Autodesk Inventor part; units mm, degrees
ref_plane "YZ Plane" through (0, 0, 0) normal (1, 0, 0) x (0, 1, 0)
ref_plane "XZ Plane" through (0, 0, 0) normal (0, 1, 0) x (-1, 0, 0)
ref_plane "XY Plane" through (0, 0, 0) normal (0, 0, 1) x (1, 0, 0)
sketch "スケッチ2" plane through (0, 0, 0) normal (0, 1, 0) x (-1, 0, 0)
  line L0 (-30, 15) -> (30, 15)
  line L1 (30, 15) -> (30, -15)
  line L2 (30, -15) -> (-30, -15)
  line L3 (-30, -15) -> (-30, 15)
  line L4 (-30, 15) -> (30, -15) construction
  line L5 (30, 15) -> (-30, -15) construction
  line L6 (27.7, -12.7) -> (27.7, 12.7)
  line L7 (27.7, 12.7) -> (-27.7, 12.7)
  line L8 (-27.7, 12.7) -> (-27.7, -12.7)
  line L9 (-27.7, -12.7) -> (27.7, -12.7)
  point P0 (0, 0)
  dimension "d0" = 60
  dimension "d1" = 30
  dimension "d2" = 2.3
extrude "押し出し1" add sketch "スケッチ2" along normal mid plane 100
sketch "スケッチ3" plane through (30, -50, -15) normal (1, 0, 0) x (0, 0, -1)
  circle A0 centre (-15, 30) radius 6
  point P0 (-15, 50)
  dimension "d5" = 12
  dimension "d6" = 20
extrude "押し出し2" cut sketch "スケッチ3" against normal blind 60
properties part number "車軸受け1"
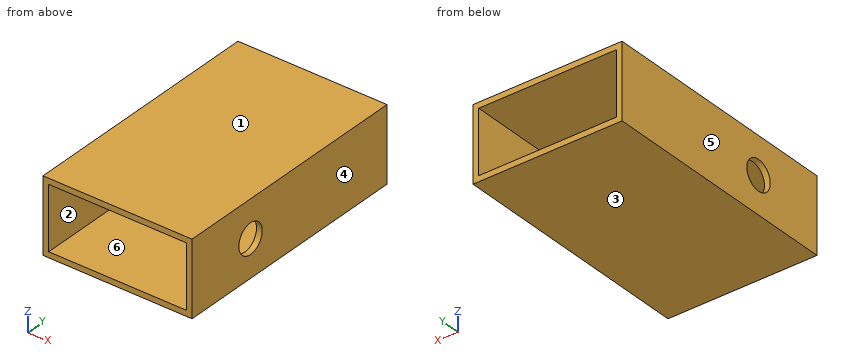
Work out the finished part from the listing and answer in its coordinate system (mm). Face numbers are marked on the shaded views. A direction names the side the tool comes from. Give positions to 0.01 mm unless a question says otherwise; leave off trailing zeros. Write each loop counter-clockwise with the first axis right and the second up, starting at its lowest first coordinate (ties: lowest second). Pieces come first, ordered by that corner, then holes. Notation, with made-up numbers: (16.25, 65.25) - (56.25, 65.25) arc R22 cw to (56.25, 73.25) - close; hole circle Ø9 at (59.5, 8). An arc over 180 degrees is marked (long way). One line per item, written item: value. Start each with the question number.
1. Find section D-D (z = 8.5). Write down the section's boundary in (x, y), then the cut area to 3 significant figures.
2. Consider probe 1 along X at (y, z) = (-36, -9); probe 2 along Y at (x, z) = (-29, 0); probe 3 along Z at (x, y) = (19, 27.5). Determine where each line is inside the solid, lowest interval first.
3. For a pull along Z with two mould halves and no side action, classify the marked faces 1, 2, 3 and 4 as +Z half, -Z half, draft (parallel to the pull), parting line (faces both ways), or undercut.
4. Find section C-C (z = 0). Write down the section's boundary in (x, y), then the cut area to 3 significant figures.
5. Find section A-A (x = 11.5). Write down the section's boundary in (y, z).
6. Find section B-B (y = -29.5). Write down the section's boundary in (x, z).
7. Given pin 1 (14 mm diameter, centred on y = -20, z = 0, fed in from +X), flat-ended and moving along its own axis, determine where the tip first touches the part or whether it passes through.
8. For the marked faces 5 and 6, determine the directions among +Z, -Z, +X, -X, +Y, -Y from which every point of the face is accessible in a straight line to the end or side of a thin tool.
Geometry results:
1. outline: (-30, -50) - (-27.7, -50) - (-27.7, 50) - (-30, 50) - close; (27.7, -50) - (30, -50) - (30, 50) - (27.7, 50) - close
1. area: 460 mm2
2. probe 1: -30 to -27.7, 27.7 to 30
2. probe 2: -50 to -26, -14 to 50
2. probe 3: -15 to -12.7, 12.7 to 15
3. face 1: +Z half
3. face 2: undercut
3. face 3: -Z half
3. face 4: draft
4. outline: (-30, -50) - (-27.7, -50) - (-27.7, -26) - (-30, -26) - close; (-30, -14) - (-27.7, -14) - (-27.7, 50) - (-30, 50) - close; (27.7, -50) - (30, -50) - (30, -26) - (27.7, -26) - close; (27.7, -14) - (30, -14) - (30, 50) - (27.7, 50) - close
4. area: 405 mm2
5. outline: (-50, -15) - (50, -15) - (50, -12.7) - (-50, -12.7) - close; (-50, 12.7) - (50, 12.7) - (50, 15) - (-50, 15) - close
6. outline: (-30, -15) - (30, -15) - (30, 15) - (-30, 15) - close; hole (-27.7, -12.7) - (27.7, -12.7) - (27.7, 12.7) - (-27.7, 12.7) - close
7. pin 1: x = 30
8. face 5: +Z, -Z, -X, +Y, -Y
8. face 6: +Y, -Y
